Autodesk Inventor part; units mm, degrees
ref_plane "YZ Plane" through (0, 0, 0) normal (1, 0, 0) x (0, 1, 0)
ref_plane "XZ Plane" through (0, 0, 0) normal (0, 1, 0) x (-1, 0, 0)
ref_plane "XY Plane" through (0, 0, 0) normal (0, 0, 1) x (1, 0, 0)
sketch "Sketch1" plane through (0, 0, 0) normal (1, 0, 0) x (0, 1, 0)
  circle A0 centre (0, 0) radius 6.477
  circle A1 centre (0, 0) radius 12.827
  dimension "connector_inner_width" = 12.954
  dimension "connector_outerdiam" = 25.654
extrude "Extrusion1" add sketch "Sketch1" along normal blind 177.8
ref_plane "Work Plane1" through (88.9, 0, 0) normal (-1, 0, 0) x (0, 0, 1)
sketch "Sketch2" plane through (0, 0, 0) normal (-1, 0, 0) x (0, 0, 1)
  circle A0 centre (0, 0) radius 12.827
  arc A1 (0, -12.827) -> (0, 12.827) centre (0, 0) ccw construction
  line L0 (-12.827, 0) -> (-12.827, 4.826)
  line L1 (-12.827, 4.826) -> (-25.527, 4.826)
  line L2 (-12.827, 4.826) -> (-12.827, 12.827) construction
  line L3 (-12.827, 0) -> (-12.827, -12.827)
  line L4 (-12.827, -12.827) -> (0, -12.827)
  line L5 (-12.827, 12.827) -> (0, 12.827)
  line L6 (-25.527, 4.826) -> (-25.527, 12.827)
  line L7 (-25.527, 12.827) -> (-12.827, 12.827)
  arc A2 (-12.827, 0) -> (0, -12.827) centre (0, 0) ccw
  arc A3 (0, 12.827) -> (-12.827, 0) centre (0, 0) ccw
  point P0 (-12.827, 0)
  point P1 (-12.827, 0)
  point P2 (0, -12.827)
  dimension "conector_tower_connection_thickness" = 4.826
  dimension "d5" = 12.7
extrude "Extrusion2" add sketch "Sketch2" against normal blind 177.8 contours A0 L0 L1 L6 L7 L5 | L4 L3 A0
sketch "Sketch3" plane through (0, 4.826, -25.527) normal (0, -1, 0) x (1, 0, 0)
  line L0 (0, 12.7) -> (177.8, 12.7)
  line L1 (0, 0) -> (177.8, 0)
  line L2 (88.9, 0) -> (88.9, 12.7) construction
  line L3 (88.9, 0) -> (88.9, 12.7) construction
  line L4 (88.9, 6.35) -> (96.52, 6.35) construction
  circle A0 centre (96.52, 6.35) radius 2.413
  line L5 (88.9, 6.35) -> (81.28, 6.35) construction
  circle A1 centre (81.28, 6.35) radius 2.413
  point P0 (0, 25.527)
  dimension "d8" = 7.62
  dimension "d9" = 4.826
extrude "Extrusion3" cut sketch "Sketch3" against normal through all
sketch "Sketch4" plane through (0, -12.827, -12.827) normal (0, 0, -1) x (-1, 0, 0)
  line L0 (0, 0) -> (-177.8, 0)
  line L1 (0, 17.653) -> (-177.8, 17.653)
  line L2 (-88.9, 8.9535) -> (-38.1, 8.9535) construction
  line L3 (-177.8, 6.35) -> (-177.8, 19.304)
  line L4 (-177.8, 12.827) -> (0, 12.827) construction
  line L5 (-88.9, 12.827) -> (-139.7, 12.827)
  circle A0 centre (-139.7, 12.827) radius 2.413
  line L6 (-88.9, 0) -> (-88.9, 17.653) construction
  circle A1 centre (-38.1, 12.827) radius 2.413
  dimension "d14" = 50.8
  dimension "d15" = 4.826
extrude "Extrusion4" cut sketch "Sketch4" against normal blind 12.7
sketch "Sketch5" plane through (0, 4.826, -25.527) normal (0, -1, 0) x (1, 0, 0)
  line L0 (0, 12.7) -> (177.8, 12.7)
  line L1 (177.8, 12.7) -> (177.8, 0)
  line L2 (0, 0) -> (177.8, 0)
  circle A0 centre (96.52, 6.35) radius 2.413
  line L3 (177.8, 0) -> (114.3, 0)
  line L4 (114.3, 0) -> (114.3, 12.7)
  line L5 (114.3, 12.7) -> (177.8, 12.7)
  point P0 (0, 25.527)
  dimension "d18" = 63.5
extrude "Extrusion5" cut sketch "Sketch5" against normal blind 12.7 contours L0 L1 L2 L4
equation "\"d6\" = connector_width"
properties part number "arm_connector"
Here's how the part is built. I have some questions about the finished solid (model axes, mm). A direction names the side the tool comes from. Give positions to 0.01 mm unless a question says otherwise; leave off trailing zeros. Write each loop counter-clockwise with the first axis right and the second up, starting at its lowest first coordinate (ties: lowest second). Pieces come first, ordered by that corner, then holes. Notation, with made-up numbers: (-36, -26) -> (2, -26) arc R14 cw to (2, 0) -> close; hole circle Ø8 at (-26.5, 38.25). An arc over 180 degrees is marked (long way). Use one line per item in the form item = value. Start each with the question number.
1. Thinking about a two-plate mould opening in X: for faces 6 (the face through (68, 12.827, -13)), 7 (the face through (177.8, 0, -8)), 8 (the face through (98.82, 8.77, -18.45)), which applies, +X half, -X half, draft (parallel to the pull), parting line (faces both ways), or undercut?
2. Imagine slicing it at D-D on x = 139.7. List the corners of the cut face in (y, z) for me.
3. Imagine slicing it at C-C on x = 96.52. List the corners of the cut face in (y, z) for me.
4. If I drill on L1, parallel to X at y = 0, z = -8; L2, parallel to X at y = 5.25, z = -19.5; L3, parallel to Y at x = 38.1, z = -7.75, over which ranges is the centre line in solid material (lowest first)?
5. Will these pins go through, and if not, where does the flat tip stop? pin 1 Ø6.5 at (y, z) = (7, -17.5) entering from +X; pin 2 Ø13 at (x, y) = (51.5, -3) entering from -Z; pin 3 Ø10 at (x, z) = (68.5, -21) entering from -Y.
6. Imagine slicing it at B-B on y = 0. List the corners of the cut face in (x, z) for me.
7. On a 3-axis mill with a long thin cutter (end or side, diameter ignored), from which of +Z, -Z, +X, -X, +Y, -Y can I reach the whole of each face in a straight line? I mean faces 1 (the face through (56, 9, -25.527)), 2 (the face through (114.3, 9, -19)), 3 (the face through (137.398, 0.725, -9.467)), 4 (the face through (56, 4.826, -19)), 5 (the face through (87.655, -1.404, 6.323)). Say none if no direction works.
8. Imagine slicing it at A-A on x = 30. List the corners of the cut face in (y, z) for me, plus the area to 3 significant figures.
Entries:
q1.face_6 = draft
q1.face_7 = +X half
q1.face_8 = undercut
q2.outline = (-12.83, -12.83) -> (-2.41, -12.83) -> (-2.41, -6.01) arc R6.48 cw (long way) to (2.41, -6.01) -> (2.41, -12.83) -> (12.83, -12.83) -> (12.83, 0) arc R12.83 ccw to (-12.83, 0) -> close
q3.outline = (-12.83, -12.83) -> (4.83, -12.83) -> (4.83, -16.76) -> (12.83, -16.76) -> (12.83, 0) arc R12.83 ccw to (-12.83, 0) -> close; (4.83, -25.53) -> (12.83, -25.53) -> (12.83, -21.59) -> (4.83, -21.59) -> close; hole circle Ø12.95 at (0, 0)
q4.L1 = 0 to 35.69, 40.51 to 137.29, 142.11 to 177.8
q4.L2 = 0 to 78.89, 83.67 to 94.13, 98.91 to 114.3
q4.L3 = -12.83 to -2.41, 2.41 to 12.83
q5.pin_1 = 114.3
q5.pin_2 = -12.83
q5.pin_3 = 4.83
q6.outline = (0, -12.83) -> (35.69, -12.83) -> (35.69, -6.48) -> (0, -6.48) -> close; (0, 6.48) -> (177.8, 6.48) -> (177.8, 12.83) -> (0, 12.83) -> close; (40.51, -12.83) -> (137.29, -12.83) -> (137.29, -6.48) -> (40.51, -6.48) -> close; (142.11, -12.83) -> (177.8, -12.83) -> (177.8, -6.48) -> (142.11, -6.48) -> close
q7.face_1 = -Z, +X, -X, +Y, -Y
q7.face_2 = -Z, +X, +Y, -Y
q7.face_3 = -Z
q7.face_4 = -Z, +X, -X, -Y
q7.face_5 = +X, -X
q8.outline = (-12.83, -12.83) -> (4.83, -12.83) -> (4.83, -25.53) -> (12.83, -25.53) -> (12.83, 0) arc R12.83 ccw to (-12.83, 0) -> close; hole circle Ø12.95 at (0, 0)
q8.area = 557 mm²
